Autodesk Inventor part; units mm, degrees
ref_plane "YZ Plane" through (0, 0, 0) normal (1, 0, 0) x (0, 1, 0)
ref_plane "XZ Plane" through (0, 0, 0) normal (0, 1, 0) x (-1, 0, 0)
ref_plane "XY Plane" through (0, 0, 0) normal (0, 0, 1) x (1, 0, 0)
sketch "Sketch1" plane through (0, 0, 0) normal (1, 0, 0) x (0, 1, 0)
  line L0 (0, 0) -> (77, 0)
  line L1 (77, 0) -> (77, -47)
  line L2 (77, -47) -> (0, -47)
  line L3 (0, -47) -> (0, 0)
  dimension "d0" = 77
  dimension "d1" = 47
extrude "Extrusion1" add sketch "Sketch1" along normal blind 6
sketch "Sketch2" plane through (6, 0, 0) normal (1, 0, 0) x (0, 0, -1)
  line L0 (47, 0) -> (47, 77)
  line L1 (47, 77) -> (47, 71)
  line L2 (47, 71) -> (41, 71)
  line L3 (41, 71) -> (41, 64.5)
  line L4 (41, 64.5) -> (47, 64.5)
  line L5 (47, 64.5) -> (47, 71)
  point P0 (0, 0)
  dimension "d4" = 6
  dimension "d5" = 6
  dimension "d6" = 6.5
extrude "Extrusion2" cut sketch "Sketch2" against normal blind 6
pattern_linear "Rectangular Pattern1" count 5 spacing 13 along (0, -1, 0) of "Extrusion2"
sketch "Sketch3" plane through (6, 0, 0) normal (1, 0, 0) x (0, 0, -1)
  line L0 (0, 77) -> (0, 0)
  line L1 (0, 77) -> (6, 77)
  line L2 (47, 77) -> (0, 77)
  line L3 (6, 77) -> (13, 77)
  line L4 (13, 77) -> (13, 71)
  line L5 (13, 71) -> (6, 71)
  line L6 (6, 71) -> (6, 77)
  line L7 (0, 0) -> (47, 0)
  line L8 (0, 0) -> (6, 0)
  line L9 (6, 0) -> (13, 0)
  line L10 (13, 0) -> (13, 6)
  line L11 (13, 6) -> (6, 6)
  line L12 (6, 6) -> (6, 0)
  dimension "d12" = 6
  dimension "d13" = 7
  dimension "d14" = 6
  dimension "d15" = 6
  dimension "d16" = 7
  dimension "d17" = 6
extrude "Extrusion3" cut sketch "Sketch3" against normal blind 6
pattern_linear "Rectangular Pattern2" count 3 spacing 14 along (0, 0, -1) of "Extrusion3"
sketch "Sketch4" plane through (6, 0, 0) normal (1, 0, 0) x (0, 0, -1)
  line L0 (47, 76.8975) -> (47, 71)
  line L1 (41, 71) -> (47, 71)
  line L2 (47, 71) -> (47, 77)
  line L3 (41, 71) -> (47, 71)
  line L4 (47, 71) -> (47, 77)
  line L5 (47, 77) -> (41, 77)
  line L6 (41, 77) -> (41, 71)
  point P0 (0, 0)
extrude "Extrusion4" cut sketch "Sketch4" against normal blind 6
properties part number "g_arm_v_3"
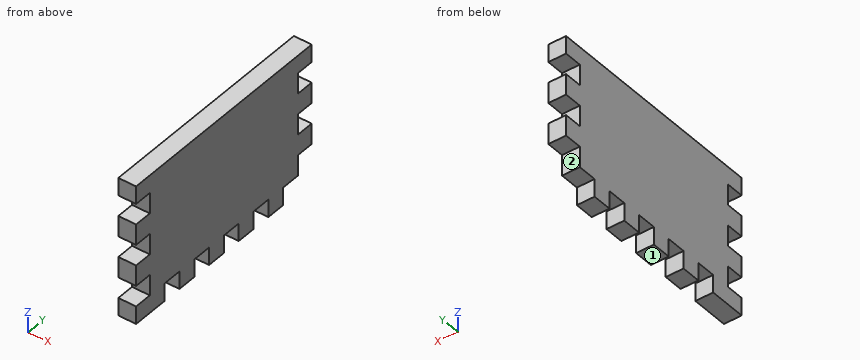
The model under review builds one solid part; all positions refer to its coordinate system, in mm. Face numbers are marked on the shaded views. A direction names the side the tool comes from. Give positions to 0.01 mm unless a question says otherwise; leave off trailing zeros. Write each loop counter-clockwise with the first axis right and the second up, starting at its lowest first coordinate (ties: lowest second). Pieces come first, ordered by that corner, then holes.
(1) Consider section A-A, the plane y = 54.5. Give the boundary of the cut face in (x, z).
(2) To check wall thickness, follow L1, parallel to Y at x = 0.55, z = -43; L2, parallel to Z at x = 0.7, y = 55; L3, parallel to Y at x = 0.95, z = -10.5. State the ranges of each line that lie inside material, in increasing order.
(3) Consider section B-B, the plane z = -11. Give the boundary of the cut face in (x, y), and give its area (3 significant figures).
(4) Tool access review of the marked faces 1 and 2: name each direction out of +Z, -Z, +X, -X, +Y, -Y from which nothing blocks a thin tool from reaching the whole face with its end or side.
(5) For P1, Ø3, axis at x = 3.5, z = -24, coming from the +Y side; P2, Ø1.5, axis at x = 4.5, y = 69, coming from the -Z side; P3, Ø3, axis at x = 2.5, z = -45, coming from the +Y side, all flat-tipped, find the tip position at first contact; note any pin that passes through.
Returned:
1. outline: (0, -41) - (6, -41) - (6, 0) - (0, 0) - close
2. L1: y = 0 to 12.5, 19 to 25.5, 32 to 38.5, 45 to 51.5, 58 to 64.5
2. L2: z = -41 to 0
2. L3: y = 6 to 71
3. outline: (0, 6) - (6, 6) - (6, 71) - (0, 71) - close
3. area: 390 mm2
4. face 1: -Z, +X, -X, +Y, -Y
4. face 2: -Z, +X, -X, +Y
5. P1: stops at y = 71
5. P2: stops at z = -41
5. P3: stops at y = 64.5
